The model under review builds one solid part; all positions refer to its coordinate system, in mm. A direction names the side the tool comes from. Coordinates: 2 decimals unless noted, no trailing zeros. Order: outer loops, then holes, each group sorted by start corner. A loop starts at its lowest first (then second) coordinate and runs counter-clockwise, first axis right, second up.
```python
from build123d import *

# Parameters (mm, degrees)
F1_DEPTH = 2
F2_R     = 6
F2_R_2   = 2.5
F2_R_3   = 5
F3_DEPTH = 1
F5_DEPTH = 8
F7_DEPTH = 6


with BuildPart() as f1:
    # F0 (on Top) → F1 (new body)
    with BuildSketch(Plane.XY):
        with BuildLine():
            Line((-36.0815, -20), (36.0815, -20))
            ThreePointArc((36.0815, -20), (50.223636, -14.142136), (56.0815, 0))
            ThreePointArc((56.0815, 0), (50.223636, 14.142136), (36.0815, 20))
            Line((36.0815, 20), (-36.0815, 20))
            ThreePointArc((-36.0815, 20), (-50.223636, 14.142136), (-56.0815, 0))
            ThreePointArc((-56.0815, 0), (-50.223636, -14.142136), (-36.0815, -20))
        make_face()
    extrude(amount=F1_DEPTH)

    # F2 (on face) → F3 (join)
    with BuildSketch(Plane.XY.offset(2)):
        with Locations((-42.0815, 7.5)):
            Circle(F2_R)
        with Locations((-42.0815, 7.5)):
            Circle(F2_R_2, mode=Mode.SUBTRACT)
        with Locations((-14.952, 12)):
            Circle(F2_R_3)
        with Locations((-14.952, 12)):
            Circle(F2_R_2, mode=Mode.SUBTRACT)
        with Locations((42.0815, 7.5)):
            Circle(F2_R)
        with Locations((42.0815, 7.5)):
            Circle(F2_R_2, mode=Mode.SUBTRACT)
        with Locations((14.952, 12)):
            Circle(F2_R_3)
        with Locations((14.952, 12)):
            Circle(F2_R_2, mode=Mode.SUBTRACT)
    extrude(amount=F3_DEPTH)

    # F4 (on face) → F5 (join)
    with BuildSketch(Plane.XY.offset(2)):
        with BuildLine():
            Line((-31.0815, -20), (0, -20))
            Line((0, -20), (31.0815, -20))
            ThreePointArc((31.0815, -20), (35.645717, -17.041549), (34.808729, -11.667169))
            Line((34.808729, -11.667169), (28.102344, -4.167169))
            ThreePointArc((28.102344, -4.167169), (26.416664, -2.935783), (24.375115, -2.5))
            Line((24.375115, -2.5), (0, -2.5))
            Line((0, -2.5), (-24.375115, -2.5))
            ThreePointArc((-24.375115, -2.5), (-26.416664, -2.935783), (-28.102344, -4.167169))
            Line((-28.102344, -4.167169), (-34.808729, -11.667169))
            ThreePointArc((-34.808729, -11.667169), (-35.645717, -17.041549), (-31.0815, -20))
        make_face()
        with BuildLine():
            Line((31.0815, -19), (0, -19))
            Line((0, -19), (-31.0815, -19))
            ThreePointArc((-31.0815, -19), (-34.732874, -16.633239), (-34.063283, -12.333735))
            Line((-34.063283, -12.333735), (-27.356898, -4.833735))
            ThreePointArc((-27.356898, -4.833735), (-26.008354, -3.848626), (-24.375115, -3.5))
            Line((-24.375115, -3.5), (0, -3.5))
            Line((0, -3.5), (24.375115, -3.5))
            ThreePointArc((24.375115, -3.5), (26.008354, -3.848626), (27.356898, -4.833735))
            Line((27.356898, -4.833735), (34.063283, -12.333735))
            ThreePointArc((34.063283, -12.333735), (34.732874, -16.633239), (31.0815, -19))
        make_face(mode=Mode.SUBTRACT)
    extrude(amount=F5_DEPTH)

    # F6 (on face) → F7 (join)
    with BuildSketch(Plane.XY.offset(2)):
        with BuildLine():
            Line((24.375115, -3.5), (-24.375115, -3.5))
            ThreePointArc((-24.375115, -3.5), (-26.008354, -3.848626), (-27.356898, -4.833735))
            Line((-27.356898, -4.833735), (-34.063283, -12.333735))
            ThreePointArc((-34.063283, -12.333735), (-34.732874, -16.633239), (-31.0815, -19))
            Line((-31.0815, -19), (31.0815, -19))
            ThreePointArc((31.0815, -19), (34.732874, -16.633239), (34.063283, -12.333735))
            Line((34.063283, -12.333735), (27.356898, -4.833735))
            ThreePointArc((27.356898, -4.833735), (26.008354, -3.848626), (24.375115, -3.5))
        make_face()
        with BuildLine():
            ThreePointArc((24.375115, -4.5), (25.600044, -4.76147), (26.611452, -5.500301))
            Line((26.611452, -5.500301), (33.317837, -13.000301))
            ThreePointArc((33.317837, -13.000301), (33.82003, -16.224929), (31.0815, -18))
            Line((31.0815, -18), (-31.0815, -18))
            ThreePointArc((-31.0815, -18), (-33.82003, -16.224929), (-33.317837, -13.000301))
            Line((-33.317837, -13.000301), (-26.611452, -5.500301))
            ThreePointArc((-26.611452, -5.500301), (-25.600044, -4.76147), (-24.375115, -4.5))
            Line((-24.375115, -4.5), (24.375115, -4.5))
        make_face(mode=Mode.SUBTRACT)
    extrude(amount=F7_DEPTH)


solid = f1.part
```
(1) Machinability: for faces 5 (the face through (0, -19, 9)), 6 (the face through (-26.39, -2.924, 5.944)), 7 (the face through (1, 20, 1)), which of the approach directions +Z, -Z, +X, -X, +Y, -Y give a long, thin tool a straight path to every point of the face, cutting with its end or side? Answer none if there is none.
A:
face 5: +Z
face 6: +Z, -X, +Y
face 7: +Z, -Z, +X, -X, +Y
(2) We need section A-A, the plane z = 7. Write out the cut boundary in (x, y).
A:
outline: (-34.81, -11.67) arc R5 ccw to (-31.08, -20) - (31.08, -20) arc R5 ccw to (34.81, -11.67) - (28.1, -4.17) arc R5 ccw to (24.38, -2.5) - (-24.38, -2.5) arc R5 ccw to (-28.1, -4.17) - close; hole (-33.32, -13) arc R3 ccw to (-31.08, -18) - (31.08, -18) arc R3 ccw to (33.32, -13) - (26.61, -5.5) arc R3 ccw to (24.38, -4.5) - (-24.38, -4.5) arc R3 ccw to (-26.61, -5.5) - close
(3) For pin 1 Ø4.5 at (x, y) = (1.5, -12) entering from +Z; pin 2 Ø1.6 at (x, z) = (-12.5, 9) entering from +Y; pin 3 Ø5.5 at (x, y) = (-13.5, 12) entering from +Z, all flat-tipped, find the tip position at first contact; note any pin that passes through.
A:
pin 1: stops at z = 2
pin 2: stops at y = -2.5
pin 3: stops at z = 3
(4) Wall thickness on probe 1 along Y at (x, z) = (-4.5, 8.5); probe 2 along Y at (x, z) = (-22, 2.5); probe 3 along Z at (x, y) = (-51, -8): over which ranges is each line inside the solid? List them lowest first.
A:
probe 1: y = -20 to -19, -3.5 to -2.5
probe 2: y = -20 to -18, -4.5 to -2.5
probe 3: z = 0 to 2
(5) We need section B-B, the plane x = -5. Write out the cut boundary in (y, z), and give its area (3 significant figures).
A:
outline: (-20, 0) - (20, 0) - (20, 2) - (-2.5, 2) - (-2.5, 10) - (-3.5, 10) - (-3.5, 8) - (-4.5, 8) - (-4.5, 2) - (-18, 2) - (-18, 8) - (-19, 8) - (-19, 10) - (-20, 10) - close
area: 108 mm2
(6) We need section C-C, the plane y = 12. Write out the cut boundary in (x, z), and give its area (3 significant figures).
A:
outline: (-52.08, 0) - (52.08, 0) - (52.08, 2) - (46.05, 2) - (46.05, 3) - (38.11, 3) - (38.11, 2) - (19.95, 2) - (19.95, 3) - (17.45, 3) - (17.45, 2) - (12.45, 2) - (12.45, 3) - (9.95, 3) - (9.95, 2) - (-9.95, 2) - (-9.95, 3) - (-12.45, 3) - (-12.45, 2) - (-17.45, 2) - (-17.45, 3) - (-19.95, 3) - (-19.95, 2) - (-38.11, 2) - (-38.11, 3) - (-46.05, 3) - (-46.05, 2) - (-52.08, 2) - close
area: 234 mm2
(7) We need section D-D, the plane x = -38. Write out the cut boundary in (y, z).
A:
outline: (-19.91, 0) - (19.91, 0) - (19.91, 2) - (11.9, 2) - (11.9, 3) - (3.1, 3) - (3.1, 2) - (-19.91, 2) - close
(8) Draft analysis for pull direction X (two halves, no side actions). For faces 1 (the face through (0, -3, 10)), 2 (the face through (0, -4.5, 5)), 3 (the face through (-35.678, -16.968, 5.944)), 4 (the face through (42, 8, 2)), state which applies: released by +X, released by -X, zero draft, split by the parting line, or undercut.
A:
face 1: zero draft
face 2: undercut
face 3: released by -X
face 4: undercut
